from build123d import *

# Parameters (mm, degrees)
F0_R     = 11
F0_R_2   = 5.5
F1_DEPTH = 6
F2_R     = 1.5
F3_DEPTH = 50.8
F4_W     = 54.249955
F4_H     = 32.60367
F5_DEPTH = 3


with BuildPart() as f1:
    # F0 (on Top) → F1 (new body)
    with BuildSketch(Plane.XY):
        with BuildLine():
            ThreePointArc((-30.408327, 1), (-19.5, 0), (-30.408327, -1))
            Line((-30.408327, -1), (-38.1, -1))
            Line((-38.1, -1), (-38.1, -8.5))
            Line((-38.1, -8.5), (-13.5, -8.5))
            Line((-13.5, -8.5), (-13.5, -13.5))
            Line((-13.5, -13.5), (13.5, -13.5))
            Line((13.5, -13.5), (13.5, -8.5))
            Line((13.5, -8.5), (38.1, -8.5))
            Line((38.1, -8.5), (38.1, 8.5))
            Line((38.1, 8.5), (13.5, 8.5))
            Line((13.5, 8.5), (13.5, 13.5))
            Line((13.5, 13.5), (-13.5, 13.5))
            Line((-13.5, 13.5), (-13.5, 8.5))
            Line((-13.5, 8.5), (-38.1, 8.5))
            Line((-38.1, 8.5), (-38.1, 1))
            Line((-38.1, 1), (-30.408327, 1))
        make_face()
        Circle(F0_R, mode=Mode.SUBTRACT)
        with Locations((25, 0)):
            Circle(F0_R_2, mode=Mode.SUBTRACT)
    extrude(amount=F1_DEPTH)

    # F2 (on face) → F3 (cut)
    with BuildSketch(Plane.XZ.offset(13.5)):
        with Locations((0, 3)):
            Circle(F2_R)
        with Locations((-33.1, 3)):
            Circle(F2_R)
    extrude(amount=-F3_DEPTH, mode=Mode.SUBTRACT)

    # F4 (on face) → F5 (cut)
    with BuildSketch(Plane.XY.offset(6)):
        with Locations((40.624977, -2.801835)):
            Rectangle(F4_W, F4_H)
    extrude(amount=-F5_DEPTH, mode=Mode.SUBTRACT)


solid = f1.part
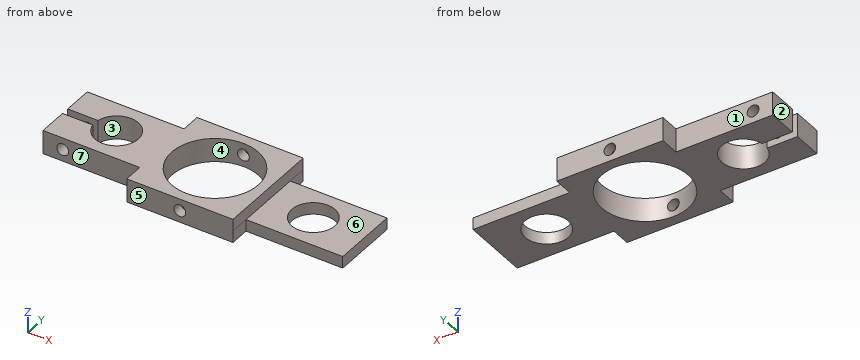
Work out the finished part from the listing and answer in its coordinate system (mm). Face numbers are marked on the shaded views. A direction names the side the tool comes from. Give positions to 0.01 mm unless a question says otherwise; leave off trailing zeros. Loops run counter-clockwise (first coordinate to the right, second up) from the corner with the lowest first, then second, coordinate; pieces in that order, holes last. Notation, with made-up numbers: (44, 13.25) -> (74, 13.25) arc R9 cw to (74, 25.25) -> close; hole circle Ø1 at (24.25, -38). An arc over 180 degrees is marked (long way). Use a Markdown table: item, result. Add a question column.
1) For a pull along Y with two mould halves and no side action, classify the marked faces 1, 2, 3 and 4 as +Y half, -Y half, draft (parallel to the pull), parting line (faces both ways), or undercut.
2) The part is cut by section D-D, the plane z = 5.25. Determine the outline of the cut face in (x, y).
3) Consider line 1 along Z through (x, y) = (-33.1, -5); line 2 along Y through (x, z) = (-25, 1.35); line 3 along Y through (x, z) = (0, 1). Determine where each line is inside the solid, lowest interval first.
4) Each of these flat-tipped pins is pushed along its axis until it touches: P1, Ø1.5, axis at y = 11, z = 2, coming from the +X side; P2, Ø3, axis at x = -34, z = 3, coming from the -Y side; P3, Ø2.5, axis at y = 12, z = 3.5, coming from the -X side; P4, Ø6.5, axis at x = 25, y = 0, coming from the +Z side. Where does it stop, or does it pass through?
5) The part is cut by section B-B, the plane y = 2. Determine the outline of the cut face in (x, z), plus the area to 3 significant figures.
6) The part is cut by section A-A, the plane x = -25. Determine the outline of the cut face in (y, z).
7) The part is cut by section C-C, the plane x = -33.1. Determine the outline of the cut face in (y, z).
8) Which of the six approach directions +Z, -Z, +X, -X, +Y, -Y give full straight-line access (tool end or side, diameter ignored) to the marked faces 5, 6 and 7?
Reported:
| question | item | result |
|---|---|---|
| 1 | face 1 | +Y half |
| 1 | face 2 | draft |
| 1 | face 3 | undercut |
| 1 | face 4 | undercut |
| 2 | outline | (-38.1, -8.5) -> (-13.5, -8.5) -> (-13.5, -13.5) -> (13.5, -13.5) -> (13.5, 13.5) -> (-13.5, 13.5) -> (-13.5, 8.5) -> (-38.1, 8.5) -> (-38.1, 1) -> (-30.41, 1) arc R5.5 cw (long way) to (-30.41, -1) -> (-38.1, -1) -> close; hole circle Ø22 at (0, 0) |
| 3 | line 1 | z = 0 to 1.5, 4.5 to 6 |
| 3 | line 2 | y = -8.5 to -5.5, 5.5 to 8.5 |
| 3 | line 3 | y = -13.5 to -11, 11 to 13.5 |
| 4 | P1 | stops at x = 13.5 |
| 4 | P2 | stops at y = -8.5 |
| 4 | P3 | stops at x = -13.5 |
| 4 | P4 | passes through |
| 5 | outline | (-38.1, 0) -> (-30.12, 0) -> (-30.12, 6) -> (-38.1, 6) -> close; (-19.88, 0) -> (-10.82, 0) -> (-10.82, 6) -> (-19.88, 6) -> close; (10.82, 0) -> (19.88, 0) -> (19.88, 3) -> (13.5, 3) -> (13.5, 6) -> (10.82, 6) -> close; (30.12, 0) -> (38.1, 0) -> (38.1, 3) -> (30.12, 3) -> close; hole circle Ø3 at (-33.1, 3) |
| 5 | area | 154 mm^2 |
| 6 | outline | (-8.5, 0) -> (-5.5, 0) -> (-5.5, 6) -> (-8.5, 6) -> close; (5.5, 0) -> (8.5, 0) -> (8.5, 6) -> (5.5, 6) -> close |
| 7 | outline | (-8.5, 0) -> (-1, 0) -> (-1, 1.5) -> (-8.5, 1.5) -> close; (-8.5, 4.5) -> (-1, 4.5) -> (-1, 6) -> (-8.5, 6) -> close; (1, 0) -> (8.5, 0) -> (8.5, 1.5) -> (1, 1.5) -> close; (1, 4.5) -> (8.5, 4.5) -> (8.5, 6) -> (1, 6) -> close |
| 8 | face 5 | +Z, -Z, +X, -X, -Y |
| 8 | face 6 | +Z, +X, +Y, -Y |
| 8 | face 7 | +Z, -Z, -X, -Y |
